from build123d import *

# Parameters (mm, degrees)
SKETCH1_R           = 3
BOSS_EXTRUDE2_DEPTH = 5


with BuildPart() as part:
    # Sketch1 → Boss-Extrude2 (new body)
    with BuildSketch(Plane.XY):
        with BuildLine():
            Line((-195.857864376, -10), (-227.161878591, -41.304014214))
            ThreePointArc((-227.161878591, -41.304014214), (-241.304014214, -41.304014214), (-241.304014214, -27.161878591))
            Line((-241.304014214, -27.161878591), (-207.071067812, 7.071067812))
            ThreePointArc((-207.071067812, 7.071067812), (-203.826834324, 9.238795325), (-200, 10))
            Line((-200, 10), (0, 10))
            ThreePointArc((0, 10), (3.826834324, 9.238795325), (7.071067812, 7.071067812))
            Line((7.071067812, 7.071067812), (107.071067812, -92.928932188))
            ThreePointArc((107.071067812, -92.928932188), (107.071067812, -107.071067812), (92.928932188, -107.071067812))
            Line((92.928932188, -107.071067812), (-4.142135624, -10))
            Line((-4.142135624, -10), (-195.857864376, -10))
        make_face()
        with Locations((-234.232946402, -34.232946402)):
            Circle(SKETCH1_R, mode=Mode.SUBTRACT)
        with Locations((100, -100)):
            Circle(SKETCH1_R, mode=Mode.SUBTRACT)
        with Locations((-160, 0)):
            Circle(SKETCH1_R, mode=Mode.SUBTRACT)
        with Locations((-40, 0)):
            Circle(SKETCH1_R, mode=Mode.SUBTRACT)
    extrude(amount=BOSS_EXTRUDE2_DEPTH)


solid = part.part
Here's how the part is built. I have some questions about the finished solid (model axes, mm). A direction names the side the tool comes from. Round coordinates to 2 decimals unless told otherwise and drop trailing zeros. Loops run counter-clockwise (first coordinate to the right, second up) from the corner with the lowest first, then second, coordinate; pieces in that order, holes last. Notation, with made-up numbers: M -10,-21 L 1,-21 A28 ccw 1,12 Z; hole C 14,86.25 d3. An arc over 180 degrees is marked long. Write each question's results on one line, items separated by ' | '. Start each with the question number.
(1) Thinking about a two-plate mould opening in Y: for faces 1 (the cylindrical face through (-237.23, -34.1, 2.46)), 2 (the flat face through (-66, -5, 5)), 3 (the flat face through (45.073, -59.215, 2.465)), which applies, pulls with the +Y half, pulls with the -Y half, needs draft (parallel to the pull), parting line crosses it, or undercut?
(2) I want a section at D-D (y = 0). Please give me the cut outline in (x, z), then the cut area to 3 significant figures.
(3) I want a section at A-A (x = -160). Please give me the cut outline in (y, z), then the cut area to 3 significant figures.
(4) I want a section at B-B (y = -100). Please give me the cut outline in (x, z), then the cut area to 3 significant figures.
(5) Will these pins go through, and if not, where does the flat tip stop? P1, Ø5, axis at x = -234.23, y = -34.23, coming from the -Z side; P2, Ø2, axis at x = -185, z = 4, coming from the -Y side; P3, Ø1.5, axis at y = -85.5, z = 4, coming from the -X side; P4, Ø1, axis at y = -80, z = 3.5, coming from the -X side.
(6) On a 3-axis mill with a long thin cutter (end or side, diameter ignored), from which of +Z, -Z, +X, -X, +Y, -Y can I reach the whole of each face in a straight line? I mean faces 4 (the flat face through (-211.29, -25.43, 2.46)), 5 (the flat face through (-66, -5, 0)). Say none if no direction works.
(7) I want a section at C-C (z = 2.2). Please give me the cut outline in (x, y).
(8) If I drill on probe 1 along Y at (x, z) = (-160, 1.4); probe 2 along X at (y, z) = (2, 1); probe 3 along Y at (x, z) = (-80.5, 0.6), over which ranges is the centre line in solid material (lowest first)? Write a range as from..to.
Solved:
1) face 1: undercut | face 2: needs draft | face 3: pulls with the -Y half
2) outline: M -214.14,0 L -163,0 L -163,5 L -214.14,5 Z; M -157,0 L -43,0 L -43,5 L -157,5 Z; M -37,0 L 14.14,0 L 14.14,5 L -37,5 Z | area: 1,080 mm²
3) outline: M -10,0 L -3,0 L -3,5 L -10,5 Z; M 3,0 L 10,0 L 10,5 L 3,5 Z | area: 70.0 mm²
4) outline: M 85.86,0 L 97,0 L 97,5 L 85.86,5 Z; M 103,0 L 110,0 L 110,5 L 103,5 Z | area: 90.7 mm²
5) P1: passes through | P2: stops at y = -10 | P3: stops at x = 70.61 | P4: stops at x = 65.36
6) face 4: +Z, -Z, -Y | face 5: -Z, +X, -X, +Y, -Y
7) outline: M -241.3,-27.16 A10 ccw -227.16,-41.3 L -195.86,-10 L -4.14,-10 L 92.93,-107.07 A10 ccw 107.07,-92.93 L 7.07,7.07 A10 ccw 0,10 L -200,10 A10 ccw -207.07,7.07 Z; hole C -234.23,-34.23 d6; hole C -160,0 d6; hole C -40,0 d6; hole C 100,-100 d6
8) probe 1: y = -10..-3, 3..10 | probe 2: x = -212.14..-162.24, -157.76..-42.24, -37.76..12.14 | probe 3: y = -10..10
